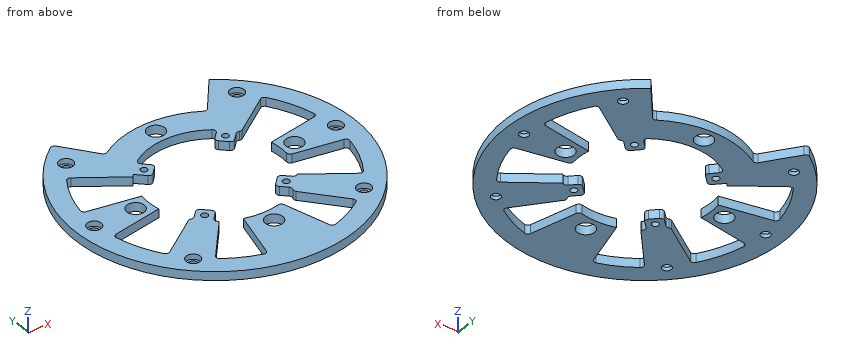
```python
from build123d import *

# Parameters (mm, degrees)
SKETCH1_R                                        = 101.6
SKETCH1_R_2                                      = 48.435876627
EXTRUDE1_DEPTH                                   = 6.35
CBORE_FOR_1_4_SOCKET_HEAD_CAP_SCREW1_D           = 6.6294
CBORE_FOR_1_4_SOCKET_HEAD_CAP_SCREW1_CBORE_D     = 10.16
CBORE_FOR_1_4_SOCKET_HEAD_CAP_SCREW1_CBORE_DEPTH = 3.81
SKETCH12_R                                       = 6.35
CUT_EXTRUDE2_DEPTH                               = 144.824345992
SKETCH13_R                                       = 2.426498152
EXTRUDE2_DEPTH                                   = 6.35
CUT_EXTRUDE3_DEPTH                               = 6.35
FILLET1_R                                        = 2.54
FILLET2_R                                        = 2.54
FILLET3_R                                        = 2.54
FILLET6_R                                        = 2.54
FILLET9_R                                        = 2.54


with BuildPart() as part:
    # Sketch1 → Extrude1 (new body)
    with BuildSketch(Plane.XY):
        Circle(SKETCH1_R)
        Circle(SKETCH1_R_2, mode=Mode.SUBTRACT)
    extrude(amount=EXTRUDE1_DEPTH)

    # CBORE for 1/4 Socket Head Cap Screw1 (through all)
    with Locations(Plane.XY.offset(6.35)):
        with Locations((62.861792847, -62.861792847), (88.9, 0), (62.861792847, 62.861792847), (-62.861792847, 62.861792847), (-88.9, 0), (-62.861792847, -62.861792847)):
            CounterBoreHole(CBORE_FOR_1_4_SOCKET_HEAD_CAP_SCREW1_D / 2, CBORE_FOR_1_4_SOCKET_HEAD_CAP_SCREW1_CBORE_D / 2, CBORE_FOR_1_4_SOCKET_HEAD_CAP_SCREW1_CBORE_DEPTH)

    # Sketch12 → Cut-Extrude2 (cut, through all)
    with BuildSketch(Plane.XY.offset(6.35)):
        with Locations((0, -58.42)):
            Circle(SKETCH12_R)
        with Locations((-58.42, 0)):
            Circle(SKETCH12_R)
        with Locations((58.42, 0)):
            Circle(SKETCH12_R)
        with Locations(Location((0, 58.42, 0), (0, 0, 180))):
            Circle(SKETCH12_R)
    extrude(amount=-CUT_EXTRUDE2_DEPTH, mode=Mode.SUBTRACT)

    # Sketch13 → Extrude2 (add)
    # profile 1 of 4: a face of its own
    with BuildSketch(Plane.XY.offset(6.35)):
        Polygon((30.067243726, -21.76182967), (44.903973325, -36.598559269), (36.598559269, -44.903973325), (21.76182967, -30.067243726), align=None)
        with Locations((29.99994, -29.99994)):
            Circle(SKETCH13_R, mode=Mode.SUBTRACT)
    # profile 2 of 4: a face of its own
    with BuildSketch(Plane.XY.offset(6.35)):
        Polygon((-30.067243726, -21.76182967), (-44.903973325, -36.598559269), (-36.598559269, -44.903973325), (-21.76182967, -30.067243726), align=None)
        with Locations((-29.99994, -29.99994)):
            Circle(SKETCH13_R, mode=Mode.SUBTRACT)
    # profile 3 of 4: a face of its own
    with BuildSketch(Plane.XY.offset(6.35)):
        Polygon((-30.067243726, 21.76182967), (-21.76182967, 30.067243726), (-36.598559269, 44.903973325), (-44.903973325, 36.598559269), align=None)
        with Locations((-29.99994, 29.99994)):
            Circle(SKETCH13_R, mode=Mode.SUBTRACT)
    # profile 4 of 4: a face of its own
    with BuildSketch(Plane.XY.offset(6.35)):
        Polygon((30.067243726, 21.76182967), (21.76182967, 30.067243726), (36.598559269, 44.903973325), (44.903973325, 36.598559269), align=None)
        with Locations((29.99994, 29.99994)):
            Circle(SKETCH13_R, mode=Mode.SUBTRACT)
    extrude(amount=-EXTRUDE2_DEPTH)

    # Sketch14 → Cut-Extrude3 (cut)
    with BuildSketch(Plane.XY.offset(6.35)):
        with BuildLine():
            Line((36.978423652, 57.45466439), (71.6832833, 101.141012966))
            Line((71.6832833, 101.141012966), (0, 148.475476712))
            Line((0, 148.475476712), (-71.6832833, 101.141012966))
            Line((-71.6832833, 101.141012966), (-38.544806548, 56.41577939))
            ThreePointArc((-38.544806548, 56.41577939), (-0.939792187, 68.319536493), (36.978423652, 57.45466439))
        make_face()
        with BuildLine():
            Line((8.652633897, -27.580853172), (23.900424698, -84.486383146))
            ThreePointArc((23.900424698, -84.486383146), (38.731626442, -78.797464115), (52.295107345, -70.52943347))
            Line((52.295107345, -70.52943347), (14.227637724, -25.162389788))
            ThreePointArc((14.227637724, -25.162389788), (11.503866682, -26.518532886), (8.652633897, -27.580853172))
        make_face()
        with BuildLine():
            Line((-71.923131973, 50.361119179), (-23.678617266, 16.579946304))
            ThreePointArc((-23.678617266, 16.579946304), (-26.705896668, 11.061944595), (-28.467103301, 5.019518375))
            Line((-28.467103301, 5.019518375), (-86.468023222, 15.246645463))
            ThreePointArc((-86.468023222, 15.246645463), (-81.118407757, 33.600344651), (-71.923131973, 50.361119179))
        make_face()
        with BuildLine():
            Line((-8.652154992, -27.581003409), (-23.900424698, -84.486383146))
            ThreePointArc((-23.900424698, -84.486383146), (-38.731626442, -78.797464115), (-52.295107345, -70.52943347))
            Line((-52.295107345, -70.52943347), (-14.229539169, -25.161314554))
            ThreePointArc((-14.229539169, -25.161314554), (-11.504638432, -26.518198083), (-8.652154992, -27.581003409))
        make_face()
        with BuildLine():
            Line((-86.468023222, -15.246645463), (-28.467103301, -5.019518375))
            ThreePointArc((-28.467103301, -5.019518375), (-26.705896668, -11.061944595), (-23.678617266, -16.579946304))
            Line((-23.678617266, -16.579946304), (-71.923131973, -50.361119179))
            ThreePointArc((-71.923131973, -50.361119179), (-81.118407757, -33.600344651), (-86.468023222, -15.246645463))
        make_face()
        with BuildLine():
            Line((23.678617266, -16.579946304), (71.923131973, -50.361119179))
            ThreePointArc((71.923131973, -50.361119179), (81.118407757, -33.600344651), (86.468023222, -15.246645463))
            Line((86.468023222, -15.246645463), (28.467103301, -5.019518375))
            ThreePointArc((28.467103301, -5.019518375), (26.705896668, -11.061944595), (23.678617266, -16.579946304))
        make_face()
        with BuildLine():
            Line((28.467103301, 5.019518375), (86.468023222, 15.246645463))
            ThreePointArc((86.468023222, 15.246645463), (81.118407757, 33.600344651), (71.923131973, 50.361119179))
            Line((71.923131973, 50.361119179), (23.678617266, 16.579946304))
            ThreePointArc((23.678617266, 16.579946304), (26.705896668, 11.061944595), (28.467103301, 5.019518375))
        make_face()
    extrude(amount=-CUT_EXTRUDE3_DEPTH, mode=Mode.SUBTRACT)

    # Fillet1
    fillet1_edges = [part.edges().sort_by_distance(p)[0] for p in [
        (-21.76182967, 30.067243726, 3.175),
        (-30.067243726, 21.76182967, 3.175),
        (21.76182967, 30.067243726, 3.175),
        (30.067243726, 21.76182967, 3.175),
        (-58.363526169, 83.1640476, 3.175),
        (52.295107345, -70.52943347, 3.175),
        (23.900424698, -84.486383146, 3.175),
        (-23.900424698, -84.486383146, 3.175),
        (-52.295107345, -70.52943347, 3.175),
        (47.700026827, -8.41080171, 3.175),
        (86.468023222, -15.246645463, 3.175),
        (71.923131973, -50.361119179, 3.175),
        (-71.923131973, -50.361119179, 3.175),
        (-86.468023222, -15.246645463, 3.175),
        (71.923131973, 50.361119179, 3.175),
        (86.468023222, 15.246645463, 3.175),
        (-86.468023222, 15.246645463, 3.175),
        (-71.923131973, 50.361119179, 3.175),
        (29.843941288, -38.149355343, 3.175),
        (30.067243726, -21.76182967, 3.175),
        (21.76182967, -30.067243726, 3.175),
        (-21.76182967, -30.067243726, 3.175),
        (-30.067243726, -21.76182967, 3.175),
    ]]
    fillet(fillet1_edges, radius=FILLET1_R)

    # Fillet2
    # the kernel refuses this fillet: 2.54 mm, written as the material it adds along each edge
    with BuildSketch(Plane(origin=(-38.149355343, -29.843941288, 6.35), x_dir=(0.7071067811865481, 0.7071067811865469, 0), z_dir=(0, 0, -1))) as fillet2_piece_1:
        with BuildLine():
            CenterArc((2.918493499, -2.54), FILLET2_R, 90, 89.954594463)
            ThreePointArc((0.378494296, -2.537987111), (0.172436891, -1.271500497), (0, 0))
            Line((0, 0), (2.918493499, 0))
        make_face()
    extrude(amount=6.35)
    # the kernel refuses this fillet: 2.54 mm, written as the material it takes off along each edge
    with BuildSketch(Plane(origin=(39.676347356, 27.781677508, 12.541699401), x_dir=(0.8191520442889919, 0.5735764363510458, 0), z_dir=(0, 0, -1))) as fillet2_2_piece_1:
        with BuildLine():
            CenterArc((2.47667976, -2.54), FILLET2_R, 90, 87.143912429)
            ThreePointArc((-0.060165151, -2.413438175), (-0.015043624, -1.207093997), (0, 0))
            Line((0, 0), (2.47667976, 0))
        make_face()
    extrude(amount=18.733398802, mode=Mode.SUBTRACT)

    # Fillet3
    # the kernel refuses this fillet: 2.54 mm, written as the material it adds along each edge
    with BuildSketch(Plane(origin=(38.149355343, -29.843941288, 6.35), x_dir=(-0.7071067811865487, 0.7071067811865462, 0), z_dir=(0, 0, -1))) as fillet3_piece_1:
        with BuildLine():
            CenterArc((2.918493499, 2.54), FILLET3_R, 180.045405537, 89.954594463)
            ThreePointArc((0.378494296, 2.537987111), (0.172436891, 1.271500497), (0, 0))
            Line((0, 0), (2.918493499, 0))
        make_face()
    extrude(amount=6.35)
    with BuildSketch(Plane(origin=(-29.843941288, 38.149355343, 6.35), x_dir=(0.8065806519344794, 0.5911240579818674, 0), z_dir=(0, 0, -1))) as fillet3_piece_2:
        with BuildLine():
            CenterArc((2.961349729, 2.538748086), FILLET3_R, 171.236815401, 100.562162322)
            Line((0.451000474, 2.925719166), (0, 0))
            ThreePointArc((0, 0), (1.52054388, -0.023873044), (3.041087761, 0))
        make_face()
    extrude(amount=6.35)
    # the kernel refuses this fillet: 2.54 mm, written as the material it takes off along each edge
    with BuildSketch(Plane(origin=(26.907852458, -40.274081253, 12.135832501), x_dir=(0.6427876096865419, -0.7660444431189757, 0), z_dir=(0, 0, -1))) as fillet3_2_piece_1:
        with BuildLine():
            CenterArc((2.314333001, -2.54), FILLET3_R, 90, 70.288335328)
            Line((-0.076827818, -1.683291217), (-0.3159439, -1.597620338))
            ThreePointArc((-0.3159439, -1.597620338), (-0.19275198, -0.605010424), (-0.252489157, -0.027662711))
            Line((-0.252489157, -0.027662711), (0, 0.254))
            Line((0, 0.254), (2.314333001, 0.254))
            Line((2.314333001, 0.254), (2.314333001, 0))
        make_face()
    extrude(amount=17.921665003, mode=Mode.SUBTRACT)
    with BuildSketch(Plane(origin=(13.709958303, -46.455044807, 12.695601727), x_dir=(-0.9660206148643552, -0.2584650298533501, 0), z_dir=(0, 0, -1))) as fillet3_2_piece_2:
        with BuildLine():
            CenterArc((2.539069601, -2.539171394), FILLET3_R, 91.463547204, 88.51545472)
            Line((-0.000930229, -2.53824052), (0, 0))
            ThreePointArc((0, 0), (1.237097807, -0.015800898), (2.474195614, 0))
        make_face()
    extrude(amount=19.041203453, mode=Mode.SUBTRACT)

    # Fillet6
    fillet6_edges = [part.edges().sort_by_distance(p)[0] for p in [
        (-29.843941288, -38.149355343, 3.175),
        (-39.676347356, -27.781677508, 3.175),
        (38.149355343, 29.843941288, 3.175),
        (29.843941288, 38.149355343, 3.175),
    ]]
    fillet(fillet6_edges, radius=FILLET6_R)

    # Fillet9
    fillet9_edges = [part.edges().sort_by_distance(p)[0] for p in [
        (-38.544806548, 56.41577939, 3.175),
        (36.978423652, 57.45466439, 3.175),
    ]]
    fillet(fillet9_edges, radius=FILLET9_R)


solid = part.part
```
For this review, take the finished solid that the model builds, in its own axes (mm). Coordinates: 2 decimals unless noted, no trailing zeros. Write each loop counter-clockwise with the first axis right and the second up, starting at its lowest first coordinate (ties: lowest second). Pieces come first, ordered by that corner, then holes. Notation, with made-up numbers: (-18.5, -23.75) - (-8.5, -23.75) arc R7 ccw to (-8.5, -15.75) - close; hole circle Ø7 at (35.5, 74.5). An arc over 180 degrees is marked (long way). Answer in a Markdown table with one row per item. Add a question column.
Q1. We need section B-B, the plane x = 77.5. State the section outline as (y, z) points.
Q2. For P1, Ø6, axis at x = -62.86, y = -62.86, coming from the +Z side, flat-tipped, find the tip position at first contact; note if it passes through.
Q3. We need section A-A, the plane y = 0. Count the separate pieces of the cut face and the enclosed holes in it, and give its area (3 significant figures).
Q4. For probe 1 along Y at (x, z) = (0.5, 2.5); probe 2 along Y at (x, z) = (0, 3.25); probe 3 along Y at (x, z) = (63, 1), list the stretches that pass through material, from the lowest coordinate up.
Answer list:
| question | item | result |
|---|---|---|
| 1 | outline | (-65.7, 0) - (-41.27, 0) - (-41.27, 6.35) - (-65.7, 6.35) - close; (-13.67, 0) - (13.67, 0) - (13.67, 6.35) - (-13.67, 6.35) - close; (41.27, 0) - (65.7, 0) - (65.7, 6.35) - (41.27, 6.35) - close |
| 2 | P1 | passes through |
| 3 | separate pieces | 6 |
| 3 | enclosed holes | 0 |
| 3 | area | 403 mm2 |
| 4 | probe 1 | y = -101.6 to -64.75, -52.09 to -48.43, 48.43 to 52.09, 64.75 to 68.32 |
| 4 | probe 2 | y = -101.6 to -64.77, -52.07 to -48.44, 48.44 to 52.07, 64.77 to 68.33 |
| 4 | probe 3 | y = -79.71 to -66.17, -59.55 to -44.11, -11.11 to -4.4, 4.4 to 11.11, 44.11 to 59.55, 66.17 to 79.71 |
